```python
from build123d import *

# Parameters (mm, degrees)
SKETCH1_W              = 36.45
SKETCH1_H              = 25.4
BOSS_EXTRUDE1_DEPTH    = 3
CUT_EXTRUDE2_START     = -3
CUT_EXTRUDE2_OUTLINE_W = 3.3
CUT_EXTRUDE2_OUTLINE_H = 5.2
CUT_EXTRUDE2_DEPTH     = 3
SKETCH2_W              = 36.45
SKETCH2_H              = 3
BOSS_EXTRUDE3_DEPTH    = 20
SKETCH5_W              = 7.3
SKETCH5_H              = 9.361177697
SKETCH5_W_2            = 3.3
SKETCH5_H_2            = 5.2
BOSS_EXTRUDE4_DEPTH    = 18
SKETCH8_W              = 29.52669185
SKETCH8_H              = 10.957410593
CUT_EXTRUDE4_DEPTH     = 47.222944791


# Read off the part's stored shape, not the designer's step: Cut-Extrude2
with BuildPart() as part:
    # Sketch1 → Boss-Extrude1 (new body)
    with BuildSketch(Plane.XY):
        with Locations((15.565968828, -4.002039549)):
            Rectangle(SKETCH1_W, SKETCH1_H)
    extrude(amount=BOSS_EXTRUDE1_DEPTH)

    # Cut-Extrude2 outline → Cut-Extrude2 (cut)
    with BuildSketch(Plane.XY.offset(3).offset(CUT_EXTRUDE2_START)):
        with Locations((24.790968828, 0.936782754)):
            Rectangle(CUT_EXTRUDE2_OUTLINE_W, CUT_EXTRUDE2_OUTLINE_H)
        with Locations((6.490968828, 0.936782754)):
            Rectangle(CUT_EXTRUDE2_OUTLINE_W, CUT_EXTRUDE2_OUTLINE_H)
    extrude(amount=CUT_EXTRUDE2_DEPTH, mode=Mode.SUBTRACT)

    # Sketch2 → Boss-Extrude3 (add)
    with BuildSketch(Plane.XY.offset(3)):
        with Locations((15.565968828, 7.197960451)):
            Rectangle(SKETCH2_W, SKETCH2_H)
        with Locations((15.565968828, -15.202039549)):
            Rectangle(SKETCH2_W, SKETCH2_H)
    extrude(amount=BOSS_EXTRUDE3_DEPTH)

    # Sketch5 → Boss-Extrude4 (add)
    # profile 1 of 2: a face of its own
    with BuildSketch(Plane.XY.offset(3)):
        with Locations((6.490968828, 1.017371602)):
            Rectangle(SKETCH5_W, SKETCH5_H)
        with Locations((6.490968828, 0.936782754)):
            Rectangle(SKETCH5_W_2, SKETCH5_H_2, mode=Mode.SUBTRACT)
    # profile 2 of 2: a face of its own
    with BuildSketch(Plane.XY.offset(3)):
        with Locations((24.790968828, 1.017371602)):
            Rectangle(SKETCH5_W, SKETCH5_H)
        with Locations((24.790968828, 0.936782754)):
            Rectangle(SKETCH5_W_2, SKETCH5_H_2, mode=Mode.SUBTRACT)
    extrude(amount=BOSS_EXTRUDE4_DEPTH)

    # Sketch8 → Cut-Extrude4 (cut, through all)
    with BuildSketch(Plane(origin=(33.790968828, 0, 0), x_dir=(0, 0, -1), z_dir=(1, 0, 0))):
        with Locations((-9.750497468, -12.749552208)):
            Rectangle(SKETCH8_W, SKETCH8_H)
    extrude(amount=-CUT_EXTRUDE4_DEPTH, mode=Mode.SUBTRACT)


solid = part.part
```
Could you check a few things on this model? Use its own coordinates, in mm. A direction names the side the tool comes from. Coordinates: 2 decimals unless noted, no trailing zeros. Write each loop counter-clockwise with the first axis right and the second up, starting at its lowest first coordinate (ties: lowest second). Pieces come first, ordered by that corner, then holes. Notation, with made-up numbers: (75, 58.5) -> (81, 58.5) arc R18 ccw to (81, 78.5) -> close; hole circle Ø7 at (10.25, 24.25). An arc over 180 degrees is marked (long way). One line per question, with ' | ' between items. Start each with the question number.
1. Will these pins go through, and if not, where does the flat tip stop? P1, Ø1.5, axis at x = 26, y = 4, coming from the -Z side; P2, Ø4.5, axis at y = -0.5, z = 14, coming from the -X side; P3, Ø3.5, axis at x = 7, z = 12, coming from the -Y side; P4, Ø4.5, axis at y = 3, z = 9, coming from the +X side.
2. Thinking about a two-plate mould opening in Y: for faces 5 (the face through (16, -7.271, 2)), 6 (the face through (4.841, 1, 10)), 7 (the face through (15, -2, 3)), which applies, pulls with the +Y half, pulls with the -Y half, needs draft (parallel to the pull), parting line crosses it, or undercut?
3. For faces 1 (the face through (28.441, 1, 12)), 2 (the face through (4, 1, 21)), 3 (the face through (2.841, 1, 12)), 4 (the face through (6, -1.663, 10)), which set-ups out of +Z, -Z, +X, -X, +Y, -Y let a thin tool reach every point of the face, with its end or its side?
4. If we section it at D-D (y = 5.25): Please give me the cut outline in (x, z).
5. If we section it at B-B (z = 12): Please give me the cut outline in (x, y), and give its area (3 significant figures).
6. If we section it at C-C (y = 0.5): Please give me the cut outline in (x, z), and give its area (3 significant figures).
7. Please list where these lines run through material, in increasing order: line 1 along X through (y, z) = (2.5, 14.25); line 2 along X through (y, z) = (5, 14); line 3 along Y through (x, z) = (8, 19.5).
8. If we section it at A-A (x = 25): Please give me the cut outline in (y, z), and give its area (3 significant figures).
Return value:
1) P1: stops at z = 0 | P2: stops at x = 2.84 | P3: stops at y = -3.66 | P4: stops at x = 28.44
2) face 5: pulls with the -Y half | face 6: undercut | face 7: needs draft
3) face 1: +Z, +X, -Y | face 2: +Z, +X, -X, -Y | face 3: +Z, -X, -Y | face 4: +Z, -Z
4) outline: (-2.66, 0) -> (33.79, 0) -> (33.79, 3) -> (28.44, 3) -> (28.44, 21) -> (21.14, 21) -> (21.14, 3) -> (10.14, 3) -> (10.14, 21) -> (2.84, 21) -> (2.84, 3) -> (-2.66, 3) -> close
5) outline: (-2.66, 5.7) -> (2.84, 5.7) -> (2.84, -3.66) -> (10.14, -3.66) -> (10.14, 5.7) -> (21.14, 5.7) -> (21.14, -3.66) -> (28.44, -3.66) -> (28.44, 5.7) -> (33.79, 5.7) -> (33.79, 8.7) -> (-2.66, 8.7) -> close; hole (4.84, -1.66) -> (8.14, -1.66) -> (8.14, 3.54) -> (4.84, 3.54) -> close; hole (23.14, -1.66) -> (26.44, -1.66) -> (26.44, 3.54) -> (23.14, 3.54) -> close | area: 212 mm²
6) outline: (-2.66, 0) -> (4.84, 0) -> (4.84, 21) -> (2.84, 21) -> (2.84, 3) -> (-2.66, 3) -> close; (8.14, 0) -> (23.14, 0) -> (23.14, 21) -> (21.14, 21) -> (21.14, 3) -> (10.14, 3) -> (10.14, 21) -> (8.14, 21) -> close; (26.44, 0) -> (33.79, 0) -> (33.79, 3) -> (28.44, 3) -> (28.44, 21) -> (26.44, 21) -> close | area: 234 mm²
7) line 1: x = 2.84 to 4.84, 8.14 to 10.14, 21.14 to 23.14, 26.44 to 28.44 | line 2: x = 2.84 to 10.14, 21.14 to 28.44 | line 3: y = -3.66 to -1.66, 3.54 to 8.7
8) outline: (-7.27, 0) -> (-1.66, 0) -> (-1.66, 21) -> (-3.66, 21) -> (-3.66, 3) -> (-7.27, 3) -> close; (3.54, 0) -> (8.7, 0) -> (8.7, 23) -> (5.7, 23) -> (5.7, 21) -> (3.54, 21) -> close | area: 167 mm²
